```python
from build123d import *

# Parameters (mm, degrees)
SM_BASE_FLANGE_1_DEPTH   = 60
SKETCH_6_R               = 13
CUT_EXTRUDE_1_DEPTH      = 5
HOLE_WIZARD_M4_1_D       = 4.8
PATTERN_CIRCULAR_1_COUNT = 4
CUT_EXTRUDE_2_DEPTH      = 5
MIRROR_3_COPY_1_DEPTH    = 5
FILLET_1_R               = 2


# Sheet-metal steps are written as plain solids
with BuildPart() as part:
    # Sketch 1 → 基体-法兰1 (new body)
    with BuildSketch(Plane.XY):
        with BuildLine():
            Line((0, 70), (0, 5.7366))
            ThreePointArc((0, 5.7366), (1.680211239, 1.680211239), (5.7366, 0))
            Line((5.7366, 0), (50, 0))
            Line((50, 0), (50, 5))
            Line((50, 5), (5.7366, 5))
            ThreePointArc((5.7366, 5), (5.215745145, 5.215745145), (5, 5.7366))
            Line((5, 5.7366), (5, 70))
            Line((5, 70), (0, 70))
        make_face()
    extrude(amount=SM_BASE_FLANGE_1_DEPTH)

    # 草图6 → 切除-拉伸1 (cut)
    with BuildSketch(Plane(origin=(5, 0, 0), x_dir=(0, 0, -1), z_dir=(1, 0, 0))):
        with Locations((-30, 45)):
            Circle(SKETCH_6_R)
    extrude(amount=-CUT_EXTRUDE_1_DEPTH, mode=Mode.SUBTRACT)

    # M4 间隙孔1 (through all)
    with Locations(Plane(origin=(5, 60.5, 45.5), x_dir=(0, 0, 1), z_dir=(1, 0, 0))):
        with Locations((0, 0)):
            hole_wizard_m4_1 = Hole(HOLE_WIZARD_M4_1_D / 2)

    # 阵列(圆周)1: M4 间隙孔1 ×4 about axis
    pattern_circular_1_axis = Axis((0, 45, 30), (1, 0, 0))
    for i in range(1, PATTERN_CIRCULAR_1_COUNT):
        add(hole_wizard_m4_1.rotate(pattern_circular_1_axis, i * 360 / PATTERN_CIRCULAR_1_COUNT), mode=Mode.SUBTRACT)

    # 草图9 → 切除-拉伸2 (cut)
    with BuildSketch(Plane(origin=(0, 5, 0), x_dir=(1, 0, 0), z_dir=(0, 1, 0))):
        with BuildLine():
            Line((41, -37), (41, -52))
            ThreePointArc((41, -52), (37.5, -55.5), (34, -52))
            Line((34, -52), (34, -37))
            ThreePointArc((34, -37), (37.5, -33.5), (41, -37))
        make_face()
    cut_extrude_2 = extrude(amount=-CUT_EXTRUDE_2_DEPTH, mode=Mode.SUBTRACT)

    # 镜向2: 切除-拉伸2 across plane
    add(cut_extrude_2.mirror(Plane(origin=(25, 0, 0), x_dir=(0, 0, 1), z_dir=(1, 0, 0))), mode=Mode.SUBTRACT)

    # 镜向3: 切除-拉伸2 across plane
    add(cut_extrude_2.mirror(Plane.XY.offset(30)), mode=Mode.SUBTRACT)

    # 镜向3 copy 1 sketch → 镜向3 copy 1 (cut)
    with BuildSketch(Plane(origin=(50, 5, 60), x_dir=(-1, 0, 0), z_dir=(0, 1, 0))):
        with BuildLine():
            Line((41, -37), (41, -52))
            ThreePointArc((41, -52), (37.5, -55.5), (34, -52))
            Line((34, -52), (34, -37))
            ThreePointArc((34, -37), (37.5, -33.5), (41, -37))
        make_face()
    extrude(amount=-MIRROR_3_COPY_1_DEPTH, mode=Mode.SUBTRACT)

    # 圆角1
    fillet_1_edges = [part.edges().sort_by_distance(p)[0] for p in [
        (50, 2.5, 60),
        (50, 2.5, 0),
        (2.5, 70, 60),
        (2.5, 70, 0),
    ]]
    fillet(fillet_1_edges, radius=FILLET_1_R)


solid = part.part
```
Part model, mm, in its own coordinate system. A direction names the side the tool comes from. Round coordinates to 2 decimals unless told otherwise and drop trailing zeros. Write each loop counter-clockwise with the first axis right and the second up, starting at its lowest first coordinate (ties: lowest second). Pieces come first, ordered by that corner, then holes. Notation, with made-up numbers: (5, -3.75) -> (20, -3.75) arc R25 cw to (20, 22.25) -> close; hole circle Ø1 at (-33, 72.5). An arc over 180 degrees is marked (long way). Return JSON: item names as keys, results as strings. Group by question number.
Q1. Saw through at D-D on x = 37.5. Write the cut outline in (y, z).
Q2. Which spindle directions (+Z, -Z, +X, -X, +Y, -Y) get a long thin tool onto all of the face, cutting with end or side? Do faces 1 (the cylindrical face through (12.6, 2.5, 26.5)), 2 (the cylindrical face through (2.465, 59.21, 16.524)), 3 (the flat face through (28, 5, 30)). Say none if no direction does.
Q3. Saw through at A-A on y = 29.5. Write the cut outline in (x, z).
Q4. Pin check, flat tips, straight feed: pin 1 (5.5 mm diameter, centred on y = 2, z = 18.5, fed in from -X); pin 2 (4 mm diameter, centred on y = 60.5, z = 45.5, fed in from +X); pin 3 (6 mm diameter, centred on y = 29.5, z = 14.5, fed in from +X); pin 4 (5 mm diameter, centred on x = 37, z = 34, fed in from +Y). Stop position of each tip, or through.
Q5. Saw through at C-C on z = 14.5. Write the cut outline in (x, y), plus the area to 3 significant figures.
Q6. Saw through at B-B on y = 45. Write the cut outline in (x, z), plus the area to 3 significant figures.
Q7. Probe L1, parallel to Z at x = 2.3, y = 29.5; L2, parallel to Y at x = 2, z = 14; L3, parallel to X at y = 9.5, z = 25.5. List the from-to ranges inside material, lowest first. Write a range as [from, to].
Q8. Mould opens along X. For faces 4 (the cylindrical face through (49.4, 2.54, 0.57)), 5 (the flat face through (4, 24, 60)), 6 (the flat face through (16, 3, 15)) say: pulls with the +X half, pulls with the -X half, needs draft (parallel to the pull), parting line crosses it, or undercut.
Answer:
{
 "1": {"outline": "(0, 0) -> (5, 0) -> (5, 4.5) -> (0, 4.5) -> close; (0, 26.5) -> (5, 26.5) -> (5, 33.5) -> (0, 33.5) -> close; (0, 55.5) -> (5, 55.5) -> (5, 60) -> (0, 60) -> close"},
 "2": {"face 1": "+Y, -Y", "face 2": "+X, -X", "face 3": "+Z, -Z, +X, +Y"},
 "3": {"outline": "(0, 0) -> (5, 0) -> (5, 12.1) -> (0, 12.1) -> close; (0, 16.9) -> (5, 16.9) -> (5, 43.1) -> (0, 43.1) -> close; (0, 47.9) -> (5, 47.9) -> (5, 60) -> (0, 60) -> close"},
 "4": {"pin 1": "x = 0.09", "pin 2": "through", "pin 3": "x = 5", "pin 4": "y = 5"},
 "5": {"outline": "(0, 5.74) arc R5.74 ccw to (5.74, 0) -> (9, 0) -> (9, 5) -> (5.74, 5) arc R0.74 cw to (5, 5.74) -> (5, 27.1) -> (0, 27.1) -> close; (0, 31.9) -> (5, 31.9) -> (5, 58.1) -> (0, 58.1) -> close; (0, 62.9) -> (5, 62.9) -> (5, 70) -> (0, 70) -> close; (16, 0) -> (34, 0) -> (34, 5) -> (16, 5) -> close; (41, 0) -> (50, 0) -> (50, 5) -> (41, 5) -> close", "area": "450 mm2"},
 "6": {"outline": "(0, 0) -> (5, 0) -> (5, 17) -> (0, 17) -> close; (0, 43) -> (5, 43) -> (5, 60) -> (0, 60) -> close", "area": "170 mm2"},
 "7": {"L1": "[0, 12.1], [16.9, 43.1], [47.9, 60]", "L2": "[1.38, 27.15], [31.85, 58.15], [62.85, 70]", "L3": "[0, 5]"},
 "8": {"face 4": "pulls with the +X half", "face 5": "needs draft", "face 6": "undercut"}
}
